CAD build for the part. Positions are in the model's coordinates, mm. Face numbers are marked on the shaded views. Coordinates: 2 decimals unless noted, no trailing zeros. Loops run counter-clockwise (first coordinate to the right, second up) from the corner with the lowest first, then second, coordinate; pieces in that order, holes last. Notation, with made-up numbers: (12, 15) -> (46, 15) arc R15 cw to (46, 23) -> close; hole circle Ø11 at (-19, 23.25). An arc over 180 degrees is marked (long way). Return JSON: item names as keys, results as strings. Group by question number.
(1) Saw through at A-A on y = 0. Write the cut outline in (x, z), then the cut area to 3 significant figures.
(2) Mould opens along X. For the marked faces 1, 2 and 3 say: pulls with the +X half, pulls with the -X half, needs draft (parallel to the pull), parting line crosses it, or undercut.
(3) Flat gauge pins, fed straight in: pin 1 Ø5 at (y, z) = (-5, 12.5) entering from -X; pin 2 Ø6 at (y, z) = (-7, 6) entering from -X; pin 3 Ø1.5 at (x, z) = (-105, 31) entering from +Y. Where does each tip first touch, or does it go through?
(4) Probe L1, parallel to Z at x = -95, y = -10; L2, parallel to Y at x = -79, z = -15.5; L3, parallel to Y at x = -89.5, z = -23.5. List the from-to ranges inside material, lowest first.
(5) Saw through at D-D on z = -9. Write the cut outline in (x, y).
(6) Saw through at C-C on x = -87. Write the cut outline in (y, z).
(7) Saw through at B-B on z = 7. Write the cut outline in (x, y), then the cut area to 3 significant figures.
```python
from build123d import *

# Parameters (mm, degrees)
CROQUIS1_R              = 50
SALIENTE_EXTRUIR1_DEPTH = 50
CROQUIS2_R              = 52
SALIENTE_EXTRUIR2_DEPTH = 10
CROQUIS3_R              = 48
CORTAR_EXTRUIR1_DEPTH   = 97
CROQUIS4_R              = 52
SALIENTE_EXTRUIR3_DEPTH = 47
CROQUIS5_R              = 45.966217712
CORTAR_EXTRUIR2_DEPTH   = 47


with BuildPart() as part:
    # Croquis1 → Saliente-Extruir1 (new body, symmetric)
    with BuildSketch(Plane.XY):
        with Locations((-84.01826484, 0)):
            Circle(CROQUIS1_R)
    extrude(amount=SALIENTE_EXTRUIR1_DEPTH, both=True)

    # Croquis2 → Saliente-Extruir2 (add)
    with BuildSketch(Plane(origin=(0, 0, -50), x_dir=(-1, 0, 0), z_dir=(0, 0, -1))):
        with Locations((84.01826484, 0)):
            Circle(CROQUIS2_R)
    extrude(amount=-SALIENTE_EXTRUIR2_DEPTH)

    # Croquis3 → Cortar-Extruir1 (cut)
    with BuildSketch(Plane.XY.offset(50)):
        with Locations((-84.01826484, 0)):
            Circle(CROQUIS3_R)
    extrude(amount=-CORTAR_EXTRUIR1_DEPTH, mode=Mode.SUBTRACT)

    # Croquis4 → Saliente-Extruir3 (add)
    with BuildSketch(Plane.XY):
        with Locations((-84.01826484, 0)):
            Circle(CROQUIS4_R)
    extrude(amount=-SALIENTE_EXTRUIR3_DEPTH)

    # Croquis5 → Cortar-Extruir2 (cut)
    with BuildSketch(Plane.XY):
        with Locations((-84.01826484, 0)):
            Circle(CROQUIS5_R)
    extrude(amount=-CORTAR_EXTRUIR2_DEPTH, mode=Mode.SUBTRACT)


solid = part.part
```
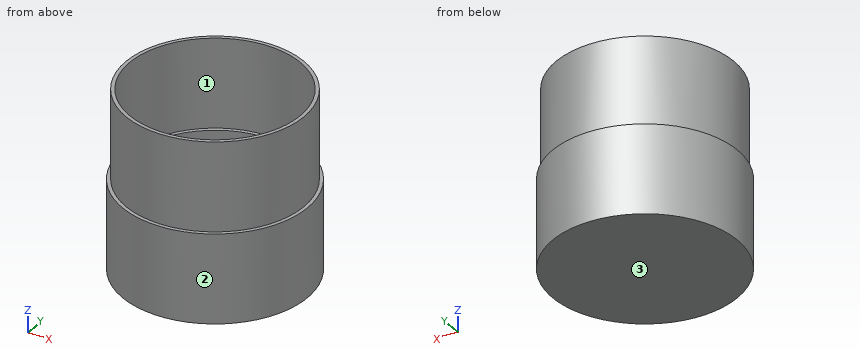
Geometry results:
{
 "1": {"outline": "(-136.02, -50) -> (-32.02, -50) -> (-32.02, 0) -> (-34.02, 0) -> (-34.02, 50) -> (-36.02, 50) -> (-36.02, 0) -> (-38.05, 0) -> (-38.05, -47) -> (-129.98, -47) -> (-129.98, 0) -> (-132.02, 0) -> (-132.02, 50) -> (-134.02, 50) -> (-134.02, 0) -> (-136.02, 0) -> close", "area": "1,080 mm²"},
 "2": {"face 1": "undercut", "face 2": "parting line crosses it", "face 3": "needs draft"},
 "3": {"pin 1": "x = -133.96", "pin 2": "x = -133.86", "pin 3": "y = 45.72"},
 "4": {"L1": "-50 to -47", "L2": "-51.76 to -45.69, 45.69 to 51.76", "L3": "-51.71 to -45.64, 45.64 to 51.71"},
 "5": {"outline": "circle Ø104 at (-84.02, 0); hole circle Ø91.93 at (-84.02, 0)"},
 "6": {"outline": "(-51.91, -50) -> (51.91, -50) -> (51.91, 0) -> (49.91, 0) -> (49.91, 50) -> (47.91, 50) -> (47.91, 0) -> (45.87, 0) -> (45.87, -47) -> (-45.87, -47) -> (-45.87, 0) -> (-47.91, 0) -> (-47.91, 50) -> (-49.91, 50) -> (-49.91, 0) -> (-51.91, 0) -> close"},
 "7": {"outline": "circle Ø100 at (-84.02, 0); hole circle Ø96 at (-84.02, 0)", "area": "616 mm²"}
}
